```python
from build123d import *

# Parameters (mm, degrees)
F0_W      = 175
F0_H      = 90
F1_DEPTH  = 55
F3_W      = 149.6
F3_H      = 64.6
F4_DEPTH  = 110
F5_W      = 149.6
F5_H      = 84.6
F6_DEPTH  = 12.7
F7_DEPTH  = 12.7
F8_R      = 1.5
F9_DEPTH  = 12.7
F10_W     = 10
F10_H     = 12.7
F10_W_2   = 20
F11_DEPTH = 10
F13_DEPTH = 137.501
F15_DEPTH = 97.501


with BuildPart() as f1:
    # F0 (on Front) → F1 (new body, symmetric)
    with BuildSketch(Plane.XZ):
        Rectangle(F0_W, F0_H)
    extrude(amount=F1_DEPTH, both=True)

    # F3 (on face) → F4 (cut)
    with BuildSketch(Plane.XZ.offset(55)):
        Rectangle(F3_W, F3_H)
    extrude(amount=-F4_DEPTH, mode=Mode.SUBTRACT)

    # F5 (on face) → F6 (cut)
    with BuildSketch(Plane.XY.offset(45)):
        Rectangle(F5_W, F5_H)
    extrude(amount=-F6_DEPTH, mode=Mode.SUBTRACT)

    # F2 (on face) → F7 (cut)
    with BuildSketch(Plane(origin=(-87.5, 0, 0), x_dir=(0, -1, 0), z_dir=(-1, 0, 0))):
        with BuildLine():
            Line((20, 18), (20, 0))
            Line((20, 0), (20, -18))
            ThreePointArc((20, -18), (20.585786, -19.414214), (22, -20))
            Line((22, -20), (33, -20))
            ThreePointArc((33, -20), (34.414214, -19.414214), (35, -18))
            Line((35, -18), (35, 0))
            Line((35, 0), (35, 18))
            ThreePointArc((35, 18), (34.414214, 19.414214), (33, 20))
            Line((33, 20), (22, 20))
            ThreePointArc((22, 20), (20.585786, 19.414214), (20, 18))
        make_face()
        with BuildLine():
            Line((-22, 20), (-33, 20))
            ThreePointArc((-33, 20), (-34.414214, 19.414214), (-35, 18))
            Line((-35, 18), (-35, 0))
            Line((-35, 0), (-35, -18))
            ThreePointArc((-35, -18), (-34.414214, -19.414214), (-33, -20))
            Line((-33, -20), (-22, -20))
            ThreePointArc((-22, -20), (-20.585786, -19.414214), (-20, -18))
            Line((-20, -18), (-20, 0))
            Line((-20, 0), (-20, 18))
            ThreePointArc((-20, 18), (-20.585786, 19.414214), (-22, 20))
        make_face()
    extrude(amount=-F7_DEPTH, mode=Mode.SUBTRACT)

    # F8 (on face) → F9 (cut)
    with BuildSketch(Plane.YZ.offset(87.5)):
        with BuildLine():
            ThreePointArc((-34, 0), (-27.5, -6.5), (-21, 0))
            Line((-21, 0), (-34, 0))
        make_face()
        with BuildLine():
            Line((-34, 0), (-21, 0))
            ThreePointArc((-21, 0), (-27.5, 6.5), (-34, 0))
        make_face()
        with BuildLine():
            Line((34, 0), (21, 0))
            ThreePointArc((21, 0), (27.5, -6.5), (34, 0))
        make_face()
        with BuildLine():
            ThreePointArc((34, 0), (27.5, 6.5), (21, 0))
            Line((21, 0), (34, 0))
        make_face()
        with Locations((-15, -15)):
            Circle(F8_R)
        with Locations((-15, 15)):
            Circle(F8_R)
        with Locations((15, 15)):
            Circle(F8_R)
        with Locations((15, -15)):
            Circle(F8_R)
    extrude(amount=-F9_DEPTH, mode=Mode.SUBTRACT)

    # F10 (on face) → F11 (join)
    with BuildSketch(Plane(origin=(0, 55, 0), x_dir=(-1, 0, 0), z_dir=(0, 1, 0))):
        with Locations((5, -38.65)):
            Rectangle(F10_W, F10_H)
        with Locations((-5, -38.65)):
            Rectangle(F10_W, F10_H)
        with Locations((-40, 38.65)):
            Rectangle(F10_W_2, F10_H)
        with Locations((40, 38.65)):
            Rectangle(F10_W_2, F10_H)
    extrude(amount=F11_DEPTH)

    # F12 (on face) → F13 (cut, through all)
    with BuildSketch(Plane.YZ.offset(50)):
        with BuildLine():
            ThreePointArc((60.927961, 39.828511), (60, 40.15), (59.072039, 39.828511))
            Line((59.072039, 39.828511), (60, 38.65))
            Line((60, 38.65), (60.927961, 39.828511))
        make_face()
        with BuildLine():
            Line((60, 38.65), (59.072039, 39.828511))
            ThreePointArc((59.072039, 39.828511), (58.5, 38.65), (59.072039, 37.471489))
            Line((59.072039, 37.471489), (60, 38.65))
        make_face()
        with BuildLine():
            Line((60.927961, 39.828511), (60, 38.65))
            Line((60, 38.65), (60.927961, 37.471489))
            ThreePointArc((60.927961, 37.471489), (61.349434, 37.994997), (61.5, 38.65))
            ThreePointArc((61.5, 38.65), (61.349434, 39.305003), (60.927961, 39.828511))
        make_face()
        with BuildLine():
            Line((60.927961, 37.471489), (60, 38.65))
            Line((60, 38.65), (59.072039, 37.471489))
            ThreePointArc((59.072039, 37.471489), (60, 37.15), (60.927961, 37.471489))
        make_face()
    extrude(amount=-F13_DEPTH, mode=Mode.SUBTRACT)

    # F14 (on face) → F15 (cut, through all)
    with BuildSketch(Plane.YZ.offset(10)):
        with BuildLine():
            ThreePointArc((60.927961, -37.471489), (60, -37.15), (59.072039, -37.471489))
            Line((59.072039, -37.471489), (60, -38.65))
            Line((60, -38.65), (60.927961, -37.471489))
        make_face()
        with BuildLine():
            Line((60, -38.65), (59.072039, -37.471489))
            ThreePointArc((59.072039, -37.471489), (58.5, -38.65), (59.072039, -39.828511))
            Line((59.072039, -39.828511), (60, -38.65))
        make_face()
        with BuildLine():
            Line((60.927961, -37.471489), (60, -38.65))
            Line((60, -38.65), (60.927961, -39.828511))
            ThreePointArc((60.927961, -39.828511), (61.349434, -39.305003), (61.5, -38.65))
            ThreePointArc((61.5, -38.65), (61.349434, -37.994997), (60.927961, -37.471489))
        make_face()
        with BuildLine():
            Line((60.927961, -39.828511), (60, -38.65))
            Line((60, -38.65), (59.072039, -39.828511))
            ThreePointArc((59.072039, -39.828511), (60, -40.15), (60.927961, -39.828511))
        make_face()
    extrude(amount=-F15_DEPTH, mode=Mode.SUBTRACT)


solid = f1.part
```
The listing builds one solid part. Answer for the finished solid, in the listing's coordinates (mm). A direction names the side the tool comes from. Coordinates: 2 decimals unless noted, no trailing zeros. Write each loop counter-clockwise with the first axis right and the second up, starting at its lowest first coordinate (ties: lowest second). Pieces come first, ordered by that corner, then holes.
Q1. Section D-D, the plane y = 27.5 is taken. Write down the section's boundary in (x, z).
Returned:
outline: (-87.5, -45) - (87.5, -45) - (87.5, -6.5) - (74.8, -6.5) - (74.8, -32.3) - (-74.8, -32.3) - (-74.8, -20) - (-87.5, -20) - close; (-87.5, 20) - (-74.8, 20) - (-74.8, 45) - (-87.5, 45) - close; (74.8, 6.5) - (87.5, 6.5) - (87.5, 45) - (74.8, 45) - close
Q2. The mould has two halves that part along Z. Classify faces 1 (the flat face through (74.8, -1, 6)), 2 (the flat face through (-1, 4, -45)), 3 (the flat face through (50, 59, 37)): released by +Z, released by -Z, zero draft, split by the parting line, or undercut.
Returned:
face 1: undercut
face 2: released by -Z
face 3: zero draft
Q3. Section C-C, the plane z = 0 is taken. Write down the section's boundary in (x, y).
Returned:
outline: (-87.5, -55) - (-74.8, -55) - (-74.8, -35) - (-87.5, -35) - close; (-87.5, -20) - (-74.8, -20) - (-74.8, 20) - (-87.5, 20) - close; (-87.5, 35) - (-74.8, 35) - (-74.8, 55) - (-87.5, 55) - close; (74.8, -55) - (87.5, -55) - (87.5, -34) - (74.8, -34) - close; (74.8, -21) - (87.5, -21) - (87.5, 21) - (74.8, 21) - close; (74.8, 34) - (87.5, 34) - (87.5, 55) - (74.8, 55) - close
Q4. Which of the six approach directions +Z, -Z, +X, -X, +Y, -Y give full straight-line access (tool end or side, diameter ignored) to faces 4 (the flat face through (10, 59, -40)), 5 (the flat face through (-1, 4, -32.3)), 6 (the flat face through (-81, 35, 0))?
Returned:
face 4: +Z, -Z, +X, +Y
face 5: +Y, -Y
face 6: -X
Q5. Section A-A, the plane x = 43.5 is taken. Write down the section's boundary in (y, z), then the cut area to 3 significant figures.
Returned:
outline: (-55, -45) - (55, -45) - (55, -32.3) - (-55, -32.3) - close; (-55, 32.3) - (-42.3, 32.3) - (-42.3, 45) - (-55, 45) - close; (42.3, 32.3) - (65, 32.3) - (65, 45) - (42.3, 45) - close; hole (60.93, 37.47) arc R1.5 ccw to (61.5, 38.65) arc R1.5 ccw to (60.93, 39.83) arc R1.5 ccw (long way) to start
area: 1,840 mm2
Q6. Section B-B, the plane z = -24.5 is taken. Write down the section's boundary in (x, y).
Returned:
outline: (-87.5, -55) - (-74.8, -55) - (-74.8, 55) - (-87.5, 55) - close; (74.8, -55) - (87.5, -55) - (87.5, 55) - (74.8, 55) - close
Q7. Given P1, Ø3, axis at y = 58.5, z = 37, coming from the -X side; P2, Ø8, axis at y = 60.5, z = 36, coming from the +X side; P3, Ø5, axis at y = 62, z = -36.5, coming from the -X side, each flat-ended and moving along its own axis, determine where each tip first touches the part or whether it passes through.
Returned:
P1: stops at x = -50
P2: stops at x = 50
P3: stops at x = -10
Q8. Find the intervals of material crossed by line 1 along Z through (x, y) = (82, 15); line 2 along X through (y, z) = (-44, 14); line 3 along Z through (x, y) = (80, -27), in increasing order.
Returned:
line 1: z = -45 to -16.5, -13.5 to 13.5, 16.5 to 45
line 2: x = -87.5 to -74.8, 74.8 to 87.5
line 3: z = -45 to -6.48, 6.48 to 45
